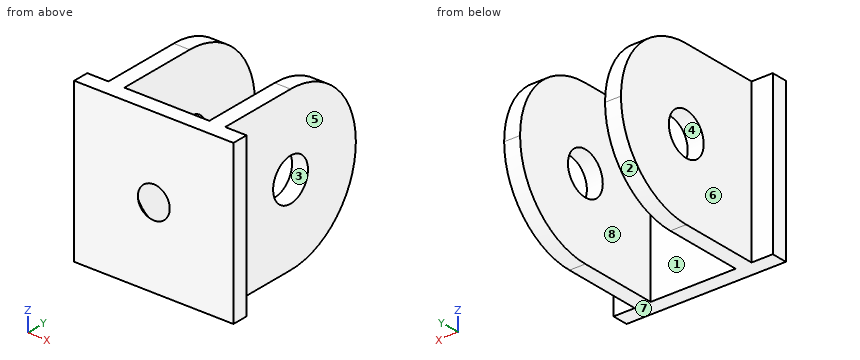
from build123d import *

# Parameters (mm, degrees)
CROQUIS1_W              = 30
CROQUIS1_H              = 30
SALIENTE_EXTRUIR1_DEPTH = 3
CROQUIS2_W              = 3
CROQUIS2_H              = 30
SALIENTE_EXTRUIR2_DEPTH = 30
REDONDEO1_R             = 15
CROQUIS3_R              = 4
CORTAR_EXTRUIR1_DEPTH   = 45.609416046
CROQUIS4_R              = 3
CORTAR_EXTRUIR2_DEPTH   = 37.742346142
CHAFL_N1_SIZE           = 3


with BuildPart() as part:
    # Croquis1 → Saliente-Extruir1 (new body)
    with BuildSketch(Plane(origin=(0, 0, 0), x_dir=(1, 0, 0), z_dir=(0, 1, 0))):
        Rectangle(CROQUIS1_W, CROQUIS1_H)
    extrude(amount=SALIENTE_EXTRUIR1_DEPTH)

    # Croquis2 → Saliente-Extruir2 (add)
    with BuildSketch(Plane(origin=(0, 3, 0), x_dir=(1, 0, 0), z_dir=(0, 1, 0))):
        with Locations((-9.5, 0)):
            Rectangle(CROQUIS2_W, CROQUIS2_H)
        with Locations((9.5, 0)):
            Rectangle(CROQUIS2_W, CROQUIS2_H)
    extrude(amount=SALIENTE_EXTRUIR2_DEPTH)

    # Redondeo1
    redondeo1_edges = [part.edges().sort_by_distance(p)[0] for p in [
        (-9.5, 33, -15),
        (9.5, 33, -15),
        (9.5, 33, 15),
        (-9.5, 33, 15),
    ]]
    fillet(redondeo1_edges, radius=REDONDEO1_R - 0.0001)  # a hair under: the kernel refuses the full size

    # Croquis3 → Cortar-Extruir1 (cut, through all)
    with BuildSketch(Plane(origin=(11, 0, 0), x_dir=(0, 0, -1), z_dir=(1, 0, 0))):
        with Locations((0, 18)):
            Circle(CROQUIS3_R)
    extrude(amount=-CORTAR_EXTRUIR1_DEPTH, mode=Mode.SUBTRACT)

    # Croquis4 → Cortar-Extruir2 (cut, through all)
    with BuildSketch(Plane(origin=(0, 3, 0), x_dir=(1, 0, 0), z_dir=(0, 1, 0))):
        with Locations(Location((0, 0, 0), (0, 0, 270))):
            Circle(CROQUIS4_R)
    extrude(amount=-CORTAR_EXTRUIR2_DEPTH, mode=Mode.SUBTRACT)

    # Chaflán1
    chafl_n1_edges = [part.edges().sort_by_distance(p)[0] for p in [
        (0, 3, -3),
    ]]
    chamfer(chafl_n1_edges, length=CHAFL_N1_SIZE - 0.0001)  # a hair under: the kernel refuses the full size


solid = part.part
Can you work these out from the model? Positions are in its coordinate system, mm. Face numbers are marked on the shaded views. A direction names the side the tool comes from. Give positions to 0.01 mm unless a question says otherwise; leave off trailing zeros. Write each loop counter-clockwise with the first axis right and the second up, starting at its lowest first coordinate (ties: lowest second). Pieces come first, ordered by that corner, then holes. Notation, with made-up numbers: M -23,55 L 27,55 A7 ccw 27,61 Z; hole C 10.25,57.25 d6. An arc over 180 degrees is marked long. Answer in a Markdown table with one row per item. Add a question column.
Item 1: We'd pull the mould along Z, two halves only. Please class the marked faces 1, 2, 3 and 4: released by +Z, released by -Z, zero draft, split by the parting line, or undercut.
Item 2: For pin 1 Ø2 at (x, z) = (13, 0.5) entering from +Y; pin 2 Ø15 at (y, z) = (13, -3.5) entering from -X; pin 3 Ø15 at (y, z) = (23, -1) entering from +X, each with a flat end and sliding along its axis, tell me the tip position at first contact or that it passes through.
Item 3: Imagine slicing it at B-B, the plane y = 30. Write out the boundary of the cut face in (x, z), plus the area to 3 significant figures.
Item 4: On a 3-axis mill with a long thin cutter (end or side, diameter ignored), from which of +Z, -Z, +X, -X, +Y, -Y can I reach the whole of each face in a straight line? I mean the marked faces 5, 6, 7 and 8. Say none if no direction works.
Item 5: Imagine slicing it at D-D, the plane y = 19.5. Write out the boundary of the cut face in (x, z).
Item 6: Please list where these lines run through material, in increasing order: L1, parallel to X at y = 28, z = 8; L2, parallel to Y at x = 9.15, z = 0; L3, parallel to Y at x = 0.5, z = 9.
Evaluation:
| question | item | result |
|---|---|---|
| 1 | face 1 | zero draft |
| 1 | face 2 | released by -Z |
| 1 | face 3 | undercut |
| 1 | face 4 | undercut |
| 2 | pin 1 | stops at y = 3 |
| 2 | pin 2 | stops at x = -11 |
| 2 | pin 3 | stops at x = 11 |
| 3 | outline | M -11,-9 L -8,-9 L -8,9 L -11,9 Z; M 8,-9 L 11,-9 L 11,9 L 8,9 Z |
| 3 | area | 108 mm² |
| 4 | face 5 | +Z, -Z, +X, +Y |
| 4 | face 6 | +Z, -Z, -X, +Y |
| 4 | face 7 | -Z, +X, -X, +Y, -Y |
| 4 | face 8 | +Z, -Z, +Y |
| 5 | outline | M -11,-14.92 L -8,-14.92 L -8,-3.71 L -11,-3.71 Z; M -11,3.71 L -8,3.71 L -8,14.92 L -11,14.92 Z; M 8,-14.92 L 11,-14.92 L 11,-3.71 L 8,-3.71 Z; M 8,3.71 L 11,3.71 L 11,14.92 L 8,14.92 Z |
| 6 | L1 | x = -11 to -8, 8 to 11 |
| 6 | L2 | y = 0 to 14, 22 to 33 |
| 6 | L3 | y = 0 to 3 |
